from build123d import *

# Parameters (mm, degrees)
SKETCH1_R           = 10
SKETCH1_R_2         = 2.5
SKETCH1_R_3         = 1.5
BOSS_EXTRUDE1_DEPTH = 3
SKETCH2_W           = 5
SKETCH2_H           = 6
CUT_EXTRUDE1_DEPTH  = 3


with BuildPart() as part:
    # Sketch1 → Boss-Extrude1 (new body)
    with BuildSketch(Plane.XY):
        Circle(SKETCH1_R)
        with Locations((0, 5)):
            Circle(SKETCH1_R_2, mode=Mode.SUBTRACT)
        Circle(SKETCH1_R_3, mode=Mode.SUBTRACT)
        with Locations((0, -5)):
            Circle(SKETCH1_R_2, mode=Mode.SUBTRACT)
    extrude(amount=BOSS_EXTRUDE1_DEPTH)

    # Sketch2 → Cut-Extrude1 (cut)
    with BuildSketch(Plane.XY.offset(3)):
        with Locations((5.5, -0.5)):
            Rectangle(SKETCH2_W, SKETCH2_H)
    extrude(amount=-CUT_EXTRUDE1_DEPTH, mode=Mode.SUBTRACT)


solid = part.part
The listing builds one solid part. Answer for the finished solid, in the listing's coordinates (mm). A direction names the side the tool comes from. Coordinates: 2 decimals unless noted, no trailing zeros. Write each loop counter-clockwise with the first axis right and the second up, starting at its lowest first coordinate (ties: lowest second). Pieces come first, ordered by that corner, then holes. Notation, with made-up numbers: (-31.75, 66) - (22.25, 66) arc R13 cw to (22.25, 77) - close; hole circle Ø5 at (54, 86). An arc over 180 degrees is marked (long way). Put each result on its own line as item: value.
1. The part is cut by section B-B on z = 1.9. Give the vertices of the cut face in (x, y), plus the area to 3 significant figures.
Answer sheet:
outline: circle Ø20 at (0, 0); hole circle Ø5 at (0, -5); hole circle Ø5 at (0, 5); hole circle Ø3 at (0, 0); hole (3, -3.5) - (8, -3.5) - (8, 2.5) - (3, 2.5) - close
area: 238 mm^2
2. The part is cut by section A-A on y = 0. Give the vertices of the cut face in (x, z).
Answer sheet:
outline: (-10, 0) - (-1.5, 0) - (-1.5, 3) - (-10, 3) - close; (1.5, 0) - (3, 0) - (3, 3) - (1.5, 3) - close; (8, 0) - (10, 0) - (10, 3) - (8, 3) - close
3. Find the intervals of material crossed by line 1 along Y through (x, z) = (0, 1.3); line 2 along X through (y, z) = (-1, 0.1); line 3 along X through (y, z) = (-1.75, 0.3), in increasing order. Write a range as from..to.
Answer sheet:
line 1: y = -10..-7.5, -2.5..-1.5, 1.5..2.5, 7.5..10
line 2: x = -9.95..-1.12, 1.12..3, 8..9.95
line 3: x = -9.85..3, 8..9.85
4. The part is cut by section D-D on x = 4. Give the vertices of the cut face in (y, z).
Answer sheet:
outline: (-9.17, 0) - (-3.5, 0) - (-3.5, 3) - (-9.17, 3) - close; (2.5, 0) - (9.17, 0) - (9.17, 3) - (2.5, 3) - close
5. A tool of negligible diameter and unlimited length cuts with its end or side. For faces 1 (the face through (5, -3.5, 2)), 2 (the face through (0, -2, 0)), from which of +Z, -Z, +X, -X, +Y, -Y can it reach the whole face along a straight path? Write none if from no direction.
Answer sheet:
face 1: +Z, -Z
face 2: -Z, +X, -X, +Y, -Y
6. Flat-ended cylindrical pins translate along their axes: pin 1 Ø10 at (x, y) = (7, 1) entering from -Z; pin 2 Ø0.9 at (x, z) = (5, 1.5) entering from +Y; pin 3 Ø1.5 at (x, z) = (7.5, 1.5) entering from +Y; pin 4 Ø4.5 at (x, y) = (0, -5) entering from -Z. Find the tip coordinate at first contact, or state that the pin passes through.
Answer sheet:
pin 1: stops at z = 0
pin 2: stops at y = 8.9
pin 3: stops at y = 7.38
pin 4: passes through
7. The part is cut by section C-C on x = 0. Give the vertices of the cut face in (y, z).
Answer sheet:
outline: (-10, 0) - (-7.5, 0) - (-7.5, 3) - (-10, 3) - close; (-2.5, 0) - (-1.5, 0) - (-1.5, 3) - (-2.5, 3) - close; (1.5, 0) - (2.5, 0) - (2.5, 3) - (1.5, 3) - close; (7.5, 0) - (10, 0) - (10, 3) - (7.5, 3) - close
8. Determine the mould class of faces 3 (the face through (0, -2, 3)), 4 (the face through (-0.33, 7.48, 1.48)), 5 (the face through (8, -1, 2)), 6 (the face through (-2.17, -9.76, 1.48)) for opening direction X: pulls with the +X half, pulls with the -X half, needs draft (parallel to the pull), parting line crosses it, or undercut.
Answer sheet:
face 3: needs draft
face 4: undercut
face 5: undercut
face 6: parting line crosses it
